Job drawing, mm, ordinate dimensions from the low corner. One solid piece. A direction names the side the tool comes from. Give positions to 0.01 mm unless a question says otherwise; leave off trailing zeros. Order: outer loops, then holes, each group sorted by start corner. A loop starts at its lowest first (then second) coordinate and runs counter-clockwise, first axis right, second up.
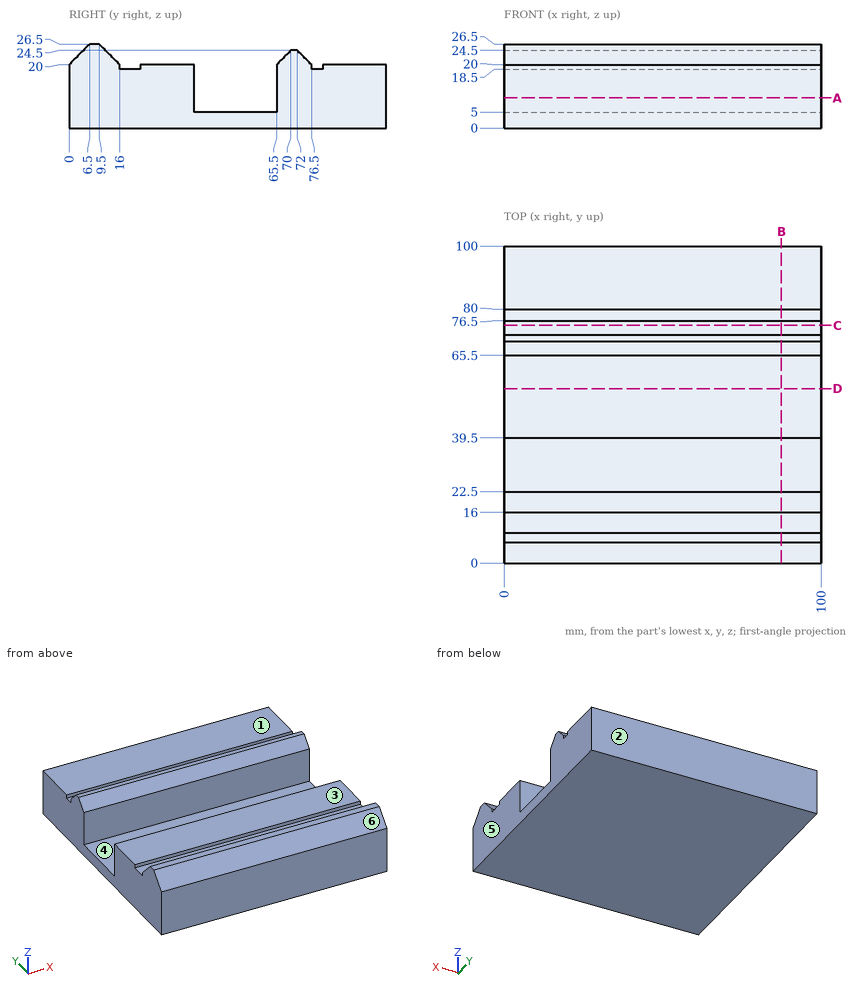
Item 1: Pull direction Y, two halves, no side cores. Call the marked faces 4, 5 and 6: released by +Y, released by -Y, zero draft, split by the parting line, or undercut.
Item 2: Drop flat-ended pins along their axis: P1, Ø1.8, axis at x = 43.5, y = 78, coming from the +Z side; P2, Ø8, axis at x = 46, y = 58.5, coming from the +Z side; P3, Ø1, axis at x = 57.5, y = 71, coming from the +Z side. Give the stop position or say it passes through.
Item 3: Band-saw the part on A-A on z = 9.5. List the corners of the cut face in (x, y).
Item 4: Drill centre lines: probe 1 along Y at (x, z) = (17, 19.25); probe 2 along Y at (x, z) = (63, 14.25); probe 3 along Y at (x, z) = (72, 23.5). Where is each one in solid material? Low to high.
Item 5: Band-saw the part on C-C on y = 75. List the corners of the cut face in (x, z).
Item 6: Band-saw the part on D-D on y = 55. List the corners of the cut face in (x, z), plus the area to 3 significant figures.
Item 7: Band-saw the part on B-B on x = 87.5. List the corners of the cut face in (y, z).
Item 8: Which spindle directions (+Z, -Z, +X, -X, +Y, -Y) get a long thin tool onto all of the face, cutting with end or side? Do the marked faces 1, 2 and 3. Say none if no direction does.
Working result:
1. face 4: undercut
1. face 5: zero draft
1. face 6: released by -Y
2. P1: stops at z = 18.5
2. P2: stops at z = 5
2. P3: stops at z = 24.5
3. outline: (0, 0) - (100, 0) - (100, 39.5) - (0, 39.5) - close; (0, 65.5) - (100, 65.5) - (100, 100) - (0, 100) - close
4. probe 1: y = 0 to 16, 22.5 to 39.5, 65.5 to 76.5, 80 to 100
4. probe 2: y = 0 to 39.5, 65.5 to 100
4. probe 3: y = 3.5 to 12.5, 69 to 73
5. outline: (0, 0) - (100, 0) - (100, 21.5) - (0, 21.5) - close
6. outline: (0, 0) - (100, 0) - (100, 5) - (0, 5) - close
6. area: 500 mm2
7. outline: (0, 0) - (100, 0) - (100, 20) - (80, 20) - (80, 18.5) - (76.5, 18.5) - (76.5, 20) - (72, 24.5) - (70, 24.5) - (65.5, 20) - (65.5, 5) - (39.5, 5) - (39.5, 20) - (22.5, 20) - (22.5, 18.5) - (16, 18.5) - (16, 20) - (9.5, 26.5) - (6.5, 26.5) - (0, 20) - close
8. face 1: +Z, +X, -X, +Y
8. face 2: +Z, -Z, +X, -X, +Y
8. face 3: +Z, +X, -X
